Source: CAD feature listing. Evaluate the final solid. Frame: model axes, mm. Face numbers are marked on the shaded views. A direction names the side the tool comes from. Give positions to 0.01 mm unless a question says otherwise; leave off trailing zeros. Order: outer loops, then holes, each group sorted by start corner. A loop starts at its lowest first (then second) coordinate and runs counter-clockwise, first axis right, second up. Notation, with made-up numbers: (53, 50.25) -> (78, 50.25) arc R5 cw to (78, 54.25) -> close; hole circle Ø3 at (42, -23.75). An arc over 180 degrees is marked (long way). Answer in a Markdown table with one row per item.
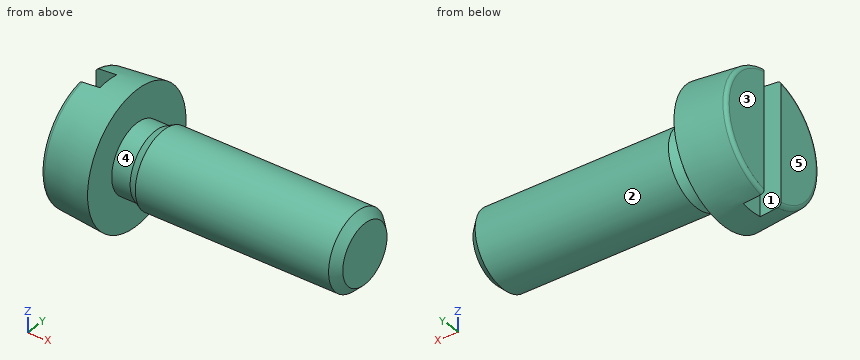
Autodesk Inventor part; units mm, degrees
ref_plane "Work Plane1" through (30.1625, 0, 0) normal (0, 0, -1) x (1, 0, 0)
ref_plane "YZ Plane" through (0, 0, 0) normal (1, 0, 0) x (0, 1, 0)
ref_plane "XZ Plane" through (0, 0, 0) normal (0, 1, 0) x (-1, 0, 0)
sketch "Sketch1" plane through (0, 0, 0) normal (0, 0, 1) x (1, 0, 0)
  line L0 (-2.6, 0) -> (12, 0)
  line L1 (12, 0) -> (12, 2)
  line L2 (12, 2) -> (1.4, 2)
  line L3 (1.4, 2) -> (0.9705, 1.7853)
  line L4 (0.9705, 1.7853) -> (0, 1.7853)
  line L5 (0, 1.7853) -> (0, 3.5)
  line L6 (-5.52, 0) -> (14.92, 0)
  line L7 (0, -0.7) -> (0, 4.2)
  line L8 (-2.6, 0) -> (-2.6, 3.2725)
  line L9 (0, 3.5) -> (-2.6, 3.2725)
  line L10 (1.4, 2) -> (0, 2) construction
  dimension "d0" = 12
  dimension "d1" = 10.6
  dimension "d2" = 0.4295
  dimension "d3" = 2.6
  dimension "d4" = 4
  dimension "d5" = 3.5705
  dimension "d9" = 7
  dimension "d10" = 5
revolve "Body" add sketch "Sketch1" angle 360 about axis through (-2.6, 0, 0) along (1, 0, 0)
sketch "Sketch2" plane through (-2.6, 0, 0) normal (-1, 0, 0) x (0, 0, 1)
  circle A0 centre (0, 0) radius 3.5
  line L0 (0, 0) -> (0, 3.2725)
  line L1 (-3.5, 0.6) -> (3.5, 0.6)
  line L2 (3.5, 0.6) -> (3.5, -0.6)
  line L3 (3.5, -0.6) -> (-3.5, -0.6)
  line L4 (-3.5, -0.6) -> (-3.5, 0.6)
  line L5 (-3.5, 0) -> (3.5, 0) construction
  line L6 (0, 0.6) -> (0, -0.6) construction
  dimension "d11" = 1.2
  dimension "d12" = 7
fillet "Fillet1" radius 0.2 1 edges at (-2.6, -3.2725, 0)
extrude "Slot" cut sketch "Sketch2" against normal blind 1.1 contours A0 L3 L1 | L2 L3 A0 | A0 L1 L2 | A0 L4 L1 | L3 L4 A0
thread "Thread"
chamfer "Chamfer1" distance 0.4294 distance2 0.4295 1 edges at (12, -2, 0) measured on face at (12, 0.6473, -0.1595)
ref_plane "Work Plane1" through (30.1625, 0, 0) normal (0, 0, -1) x (1, 0, 0)
equation "\"d11\" = SBR"
equation "\"d12\" = KOD"
equation "\"d19\" = STI"
equation "\"d14\" = RR"
equation "\"d15\" = GEL"
equation "\"d17\" = -0.5 * SPD + 0.5 * GD"
equation "\"d0\" = NLG"
equation "\"d1\" = GEL"
equation "\"d3\" = KOH"
equation "\"d4\" = GD"
equation "\"d5\" = BDM"
equation "\"d9\" = KOD"
equation "\"d10\" = KEWI"
equation "\"GD\" = NND"
equation "\"NLG\" = 12"
equation "\"GEL\" = 10.6"
equation "\"KOD\" = 7"
equation "\"KOH\" = 2.6"
equation "\"GAL\" = 0.61345 * PTC"
equation "\"SPD\" = NND - 1.2269 * PTC"
equation "\"BDM\" = 3.5705"
equation "\"GUL\" = 0.61345 * PTC"
equation "\"RR\" = 0.2"
equation "\"SBR\" = 1.2"
equation "\"STI\" = 1.1"
equation "\"KEWI\" = 5deg"
equation "\"PTC\" = 0.7"
equation "\"THREADDIA\" = 4"
equation "\"TOA\" = 30deg"
equation "\"NND\" = 4"
equation "\"GD1\" = THREADDIA - 1.2269 * PTC"
properties part number "ISO 1207 - M4 x 12" material "Stainless Steel, 440C"
(1) Section query D-D (x = -1). Return the cut outline in (y, z) (1 decimal), plus the area to 3 significant figures.
A:
| item | result |
|---|---|
| outline | circle Ø6.8 at (0, 0) |
| area | 36.6 mm^2 |
(2) Section query B-B (z = 0). Return the cut outline in (x, y).
A:
| item | result |
|---|---|
| outline | (-2.6, -3.09) arc R0.2 ccw to (-2.42, -3.29) -> (0, -3.5) -> (0, -1.79) -> (0.97, -1.79) -> (1.4, -2) -> (11.57, -2) -> (12, -1.57) -> (12, 1.57) -> (11.57, 2) -> (1.4, 2) -> (0.97, 1.79) -> (0, 1.79) -> (0, 3.5) -> (-2.42, 3.29) arc R0.2 ccw to (-2.6, 3.09) -> (-2.6, 0.6) -> (-1.5, 0.6) -> (-1.5, -0.6) -> (-2.6, -0.6) -> close |
(3) Ray query, probe 1 along X at (y, z) = (-2, 2); probe 2 along Z at (x, y) = (0.75, 0); probe 3 along Z at (x, y) = (6.5, 0). Return the intervals inside material, ascending.
A:
| item | result |
|---|---|
| probe 1 | x = -2.6 to 0 |
| probe 2 | z = -1.79 to 1.79 |
| probe 3 | z = -2 to 2 |
(4) Access query for the marked faces 4 and 5. Directions: +Z, -Z, +X, -X, +Y, -Y. A direction counts if a zero-diameter tool reaches every point of the face in a straight line with its end or side. Return the directions, or none.
A:
| item | result |
|---|---|
| face 4 | none |
| face 5 | +Z, -Z, -X, +Y, -Y |
(5) Section query A-A (y = 0). Return the cut outline in (x, z), plus the area to 3 significant figures.
A:
| item | result |
|---|---|
| outline | (-1.5, -3.37) -> (0, -3.5) -> (0, -1.79) -> (0.97, -1.79) -> (1.4, -2) -> (11.57, -2) -> (12, -1.57) -> (12, 1.57) -> (11.57, 2) -> (1.4, 2) -> (0.97, 1.79) -> (0, 1.79) -> (0, 3.5) -> (-1.5, 3.37) -> close |
| area | 57.6 mm^2 |
(6) Section query C-C (x = 8.5). Return the cut outline in (y, z).
A:
| item | result |
|---|---|
| outline | circle Ø4 at (0, 0) |
(7) First-contact query: pin 1 Ø3 at (x, z) = (6, 0.5) entering from +Y; pin 2 Ø0.9 at (x, z) = (-2, -0.5) entering from -Y; pin 3 Ø3 at (x, z) = (6.5, 0.5) entering from -Y. Flat tips, straight axial feed; report the tip coordinate or a pass-through.
A:
| item | result |
|---|---|
| pin 1 | stops at y = 2 |
| pin 2 | stops at y = -3.35 |
| pin 3 | stops at y = -2 |
(8) Pull-direction query (Y, two-part tool) for the marked faces 1, 2 and 3; classes: +Y half, -Y half, draft (parallel to the pull), parting line (faces both ways), or undercut.
A:
| item | result |
|---|---|
| face 1 | undercut |
| face 2 | parting line |
| face 3 | draft |
